Verification items for this drawing (mm, ordinates from the low corner). A direction names the side the tool comes from. Round coordinates to 2 decimals unless told otherwise and drop trailing zeros. Loops run counter-clockwise (first coordinate to the right, second up) from the corner with the lowest first, then second, coordinate; pieces in that order, holes last. Notation, with made-up numbers: M 46.5,67 L 55.5,67 A18 ccw 55.5,73 Z; hole C 18,39.5 d1. An arc over 180 degrees is marked long. Write item = value, one per line.
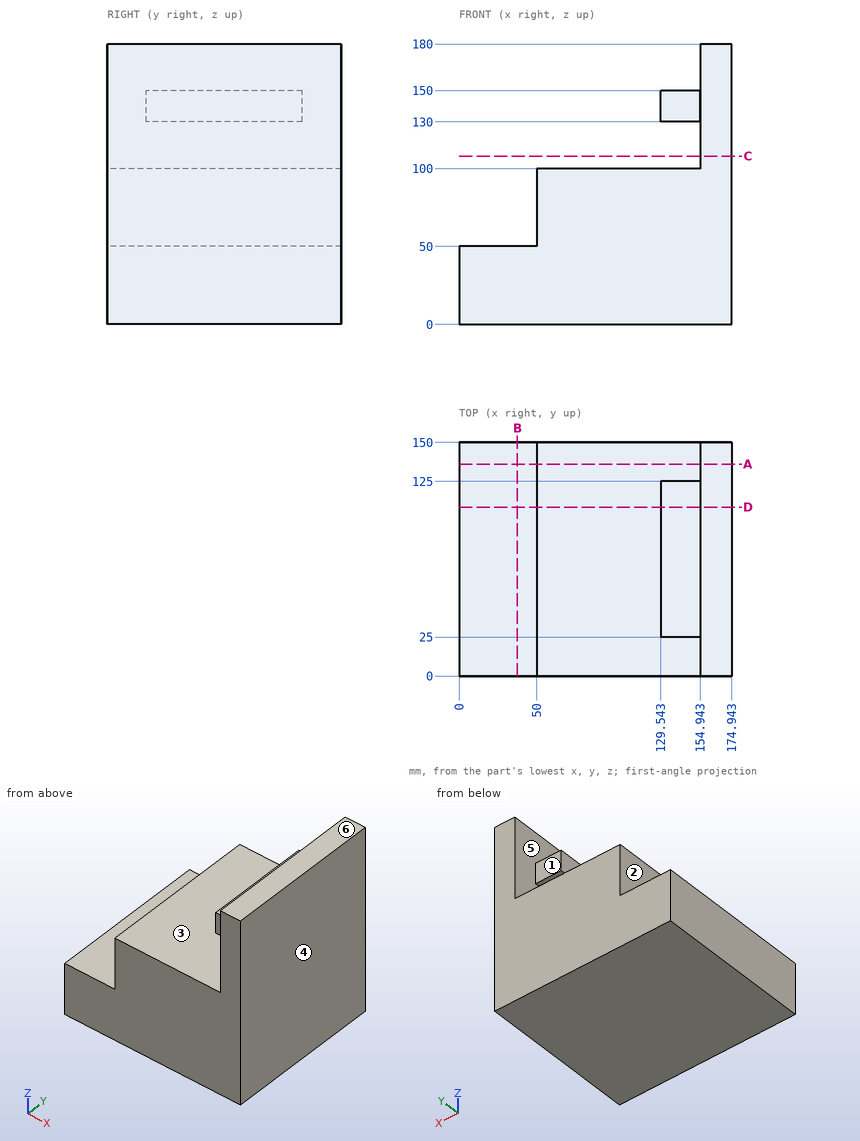
(1) Tool access check on the marked faces 1, 2 and 3. Record the directions out of +Z, -Z, +X, -X, +Y, -Y that give a thin tool (end or side, any length) a straight path to the whole face; none if there is none.
Result set:
face_1 = +Z, -X, +Y
face_2 = +Z, -X, +Y, -Y
face_3 = -X, +Y, -Y
(2) Sectioned sample at B-B on x = 37.5. Record the cut outline in (y, z).
Result set:
outline = M 0,0 L 150,0 L 150,50 L 0,50 Z
(3) Release check for a two-part mould opening along Z. For the marked faces 4, 5 and 6 record: released by +Z, released by -Z, zero draft, split by the parting line, or undercut.
Result set:
face_4 = zero draft
face_5 = undercut
face_6 = released by +Z
(4) Depth check by flat-ended pin: pin 1 Ø8 at (y, z) = (115, 61.5) entering from -X; pin 2 Ø6 at (y, z) = (64, 140.5) entering from -X; pin 3 Ø2 at (x, y) = (100.5, 17.5) entering from +Z. Enter the tip coordinate at first touch or a pass-through.
Result set:
pin_1 = 50
pin_2 = 129.54
pin_3 = 100
(5) Sectioned sample at D-D on y = 108.5. Record the cut outline in (x, z), then the cut area to 3 significant figures.
Result set:
outline = M 0,0 L 174.94,0 L 174.94,180 L 154.94,180 L 154.94,150 L 129.54,150 L 129.54,130 L 154.94,130 L 154.94,100 L 50,100 L 50,50 L 0,50 Z
area = 17,100 mm2
(6) Sectioned sample at A-A on y = 136. Record the cut outline in (x, z), then the cut area to 3 significant figures.
Result set:
outline = M 0,0 L 174.94,0 L 174.94,180 L 154.94,180 L 154.94,100 L 50,100 L 50,50 L 0,50 Z
area = 16,600 mm2
(7) Material ranges on line 1 along Z through (x, y) = (152.5, 121); line 2 along Z through (x, y) = (60.5, 37); line 3 along X through (y, z) = (19, 141.5), recorded low to high. Write a range as from..to.
Result set:
line_1 = 0..100, 130..150
line_2 = 0..100
line_3 = 154.94..174.94
(8) Sectioned sample at C-C on z = 108. Record the cut outline in (x, y).
Result set:
outline = M 154.94,0 L 174.94,0 L 174.94,150 L 154.94,150 Z
